from build123d import *

# Parameters (mm, degrees)
SKETCH_1_R          = 4.1
SKETCH_1_R_2        = 1.5
EXTRUDE_1_DEPTH     = 8.4
SKETCH_2_W          = 10.2
SKETCH_2_H          = 10.2
CUT_EXTRUDE_1_DEPTH = 5


with BuildPart() as part:
    # ｽｹｯﾁ1 → ﾎﾞｽ - 押し出し1 (new body)
    with BuildSketch(Plane(origin=(0, 0, 0), x_dir=(1, 0, 0), z_dir=(0, 1, 0))):
        with BuildLine():
            Line((-90.755581693, -47.201953746), (29.244418307, -19.748139436))
            ThreePointArc((29.244418307, -19.748139436), (34.834131004, -16.232897902), (37.014221558, -10))
            Line((37.014221558, -10), (37.014221558, 10))
            ThreePointArc((37.014221558, 10), (34.834131004, 16.232897902), (29.244418307, 19.748139436))
            Line((29.244418307, 19.748139436), (-90.755581693, 47.201953746))
            ThreePointArc((-90.755581693, 47.201953746), (-99.218676344, 45.273723756), (-102.985778442, 37.45381431))
            Line((-102.985778442, 37.45381431), (-102.985778442, -37.45381431))
            ThreePointArc((-102.985778442, -37.45381431), (-99.218676344, -45.273723756), (-90.755581693, -47.201953746))
        make_face()
        with Locations(Location((-82.985778442, 0, 0), (0, 0, 270))):
            Circle(SKETCH_1_R, mode=Mode.SUBTRACT)
        with Locations(Location((27.014221558, 0, 0), (0, 0, 270))):
            Circle(SKETCH_1_R, mode=Mode.SUBTRACT)
        with Locations(Location((-87.985778442, 35, 0), (0, 0, 270))):
            Circle(SKETCH_1_R_2, mode=Mode.SUBTRACT)
        with Locations(Location((-87.985778442, -35, 0), (0, 0, 270))):
            Circle(SKETCH_1_R_2, mode=Mode.SUBTRACT)
    extrude(amount=EXTRUDE_1_DEPTH)

    # ｽｹｯﾁ2 → ｶｯﾄ - 押し出し1 (cut)
    with BuildSketch(Plane.XZ):
        with Locations((-87.985778442, 35)):
            Rectangle(SKETCH_2_W, SKETCH_2_H)
        with Locations((-87.985778442, -35)):
            Rectangle(SKETCH_2_W, SKETCH_2_H)
    extrude(amount=-CUT_EXTRUDE_1_DEPTH, mode=Mode.SUBTRACT)


solid = part.part
The model under review builds one solid part; all positions refer to its coordinate system, in mm. A direction names the side the tool comes from. Coordinates: 2 decimals unless noted, no trailing zeros. Loops run counter-clockwise (first coordinate to the right, second up) from the corner with the lowest first, then second, coordinate; pieces in that order, holes last. Notation, with made-up numbers: M 34,65 L 43,65 A13 ccw 43,72 Z; hole C 86.5,82.5 d8. An arc over 180 degrees is marked long. Put each result on its own line as item: value. Start each with the question number.
Q1. Add section A-A (z = 0). Write out the cut boundary in (x, y).
Q2. Add section D-D (x = 20.5). Write out the cut boundary in (y, z).
Q3. The part is to be moulded in two halves that separate along Z. For faces 3 (the flat face through (-31.6, 4.14, 33.67)), 4 (the flat face through (-93.086, 2, 35)), 5 (the flat face through (-102.986, 4, -1)), say which applies: +Z half, -Z half, draft (parallel to the pull), parting line (faces both ways), or undercut.
Q4. Clearance check with flat-ended pins moving along their axes: pin 1 (1.5 mm diameter, centred on x = -86, y = 3.5, fed in from -Z); pin 2 (3 mm diameter, centred on x = -87, z = -34, fed in from -Y); pin 3 (2.5 mm diameter, centred on x = -88.5, y = 3.5, fed in from +Z). State where each tip first meets the part, or that it passes through.
Q5. Add section B-B (y = 2.75). Write out the cut boundary in (x, z), and give its area (3 significant figures).
Q6. Add section C-C (z = 35). Write out the cut boundary in (x, y).
Q7. For faces 1 (the flat face through (-82.886, 2, 35)), 2 (the flat face through (-50, 0, -1)), list the 3-axis set-ups (+Z, -Z, +X, -X, +Y, -Y) from which the entire face can be reached by the end or side of a thin tool; tool diameter is ignored.
Q8. Wall thickness on line 1 (X direction, y = 2.25, z = 0); line 2 (X direction, y = 3, z = -1); line 3 (Z direction, x = 17, y = 3): over which ranges is each line inside the solid? List them lowest first.
Answers:
1. outline: M -102.99,0 L -87.09,0 L -87.09,8.4 L -102.99,8.4 Z; M -78.89,0 L 22.91,0 L 22.91,8.4 L -78.89,8.4 Z; M 31.11,0 L 37.01,0 L 37.01,8.4 L 31.11,8.4 Z
2. outline: M 0,-21.75 L 8.4,-21.75 L 8.4,21.75 L 0,21.75 Z
3. face 3: +Z half
3. face 4: undercut
3. face 5: draft
4. pin 1: stops at z = -46.29
4. pin 2: stops at y = 5
4. pin 3: stops at z = 46.97
5. outline: M -102.99,-37.45 A10 ccw -90.76,-47.2 L 29.24,-19.75 A10 ccw 37.01,-10 L 37.01,10 A10 ccw 29.24,19.75 L -90.76,47.2 A10 ccw -102.99,37.45 Z; hole M -93.09,-40.1 L -82.89,-40.1 L -82.89,-29.9 L -93.09,-29.9 Z; hole M -93.09,29.9 L -82.89,29.9 L -82.89,40.1 L -93.09,40.1 Z; hole C -82.99,0 d8.2; hole C 27.01,0 d8.2
5. area: 9,110 mm^2
6. outline: M -102.99,0 L -93.09,0 L -93.09,5 L -89.49,5 L -89.49,8.4 L -102.99,8.4 Z; M -86.49,5 L -82.89,5 L -82.89,0 L -37.42,0 L -37.42,8.4 L -86.49,8.4 Z
7. face 1: -Y
7. face 2: +Z, -Z, +X, -X, -Y
8. line 1: x = -102.99 to -87.09, -78.89 to 22.91, 31.11 to 37.01
8. line 2: x = -102.99 to -86.96, -79.01 to 23.04, 30.99 to 37.01
8. line 3: z = -22.55 to 22.55
